Build history of the part. All positions in model axes, mm. A direction names the side the tool comes from. Give positions to 0.01 mm unless a question says otherwise; leave off trailing zeros. Order: outer loops, then holes, each group sorted by start corner. A loop starts at its lowest first (then second) coordinate and runs counter-clockwise, first axis right, second up. Notation, with made-up numbers: M 64.5,43.25 L 74.5,43.25 A5 cw 74.5,51.25 Z; hole C 44,80.5 d9. An arc over 180 degrees is marked long. Use CSV: the item, a comma, the result in double quotes. Start each with the question number.
Item 1: Band-saw the part on C-C on y = 3.5. Write the cut outline in (x, z), plus the area to 3 significant figures.
Item 2: Band-saw the part on D-D on x = -10. Write the cut outline in (y, z), plus the area to 3 significant figures.
Item 3: Band-saw the part on B-B on x = 5. Write the cut outline in (y, z), plus the area to 3 significant figures.
Item 4: Two-plate mould, pull along X, no slides. Class faces 1 (the flat face through (0, 11, 2)), 2 (the cylindrical face through (-10.55, -2.97, 7.44)), 3 (the flat face through (11.45, 0, 4)): pulls with the +X half, pulls with the -X half, needs draft (parallel to the pull), parting line crosses it, or undercut.
Item 5: Pin check, flat tips, straight feed: P1, Ø2.5, axis at x = 4.5, y = 10.5, coming from the +Z side; P2, Ø5.5, axis at x = 4.5, y = 11, coming from the -Z side; P3, Ø0.6, axis at x = 5, z = 7.5, coming from the +Y side. Stop position of each tip, or through.
Item 6: Wall check: line 1 along X through (y, z) = (2.25, 5); line 2 along X through (y, z) = (-2.5, 5.25); line 3 along X through (y, z) = (-4.5, 5.5). Give the ranges that are in metal, low to high.
Item 7: Which spindle directions (+Z, -Z, +X, -X, +Y, -Y) get a long thin tool onto all of the face, cutting with end or side? Do faces 4 (the flat face through (11.65, 0, 4)), 5 (the flat face through (0, -14.25, 4)), 6 (the flat face through (0, 11, 6.3)). Say none if no direction does.
Item 8: Band-saw the part on A-A on z = 4.25. Write the cut outline in (x, y), plus the area to 3 significant figures.
from build123d import *

# Parameters (mm, degrees)
EXTRUDE_1_DEPTH     = 14.25
CUT_EXTRUDE_START   = -12.229513
CUT_EXTRUDE_1_DEPTH = 24.459026


with BuildPart() as part:
    # Эскиз1 → Бобышка-Вытянуть1 (new, symmetric)
    with BuildSketch(Plane(origin=(0, 0, 0), x_dir=(1, 0, 0), z_dir=(0, 1, 0))):
        with BuildLine():
            Line((-9.25, 0), (9.25, 0))
            ThreePointArc((9.25, 0), (11.371320344, -0.878679656), (12.25, -3))
            Line((12.25, -3), (12.25, -5))
            ThreePointArc((12.25, -5), (11.95, -5.3), (11.65, -5))
            Line((11.65, -5), (11.65, -3.1))
            ThreePointArc((11.65, -3.1), (11.55, -3), (11.45, -3.1))
            Line((11.45, -3.1), (11.45, -5.3))
            ThreePointArc((11.45, -5.3), (10.571320344, -7.421320344), (8.45, -8.3))
            Line((8.45, -8.3), (-8.45, -8.3))
            ThreePointArc((-8.45, -8.3), (-10.571320344, -7.421320344), (-11.45, -5.3))
            Line((-11.45, -5.3), (-11.45, -3.1))
            ThreePointArc((-11.45, -3.1), (-11.55, -3), (-11.65, -3.1))
            Line((-11.65, -3.1), (-11.65, -5))
            ThreePointArc((-11.65, -5), (-11.95, -5.3), (-12.25, -5))
            Line((-12.25, -5), (-12.25, -3))
            ThreePointArc((-12.25, -3), (-11.371320344, -0.878679656), (-9.25, 0))
        make_face()
    extrude(amount=EXTRUDE_1_DEPTH, both=True)

    # Эскиз2 → Вырез-Вытянуть1 (cut)
    with BuildSketch(Plane(origin=(0, 0, 0), x_dir=(0, 0, -1), z_dir=(1, 0, 0)).offset(CUT_EXTRUDE_START)):
        with BuildLine():
            Line((-6.3, 13.6), (-6.3, 8.4))
            ThreePointArc((-6.3, 8.4), (-6.490380592, 7.940380592), (-6.95, 7.75))
            Line((-6.95, 7.75), (-7.65, 7.75))
            ThreePointArc((-7.65, 7.75), (-8.109619408, 7.559619408), (-8.3, 7.1))
            Line((-8.3, 7.1), (-8.3, 14.25))
            Line((-8.3, 14.25), (-8.3, 15.25))
            Line((-8.3, 15.25), (0, 15.25))
            Line((0, 15.25), (0, 7.1))
            ThreePointArc((0, 7.1), (-0.190380592, 7.559619408), (-0.65, 7.75))
            Line((-0.65, 7.75), (-1.35, 7.75))
            ThreePointArc((-1.35, 7.75), (-1.809619408, 7.940380592), (-2, 8.4))
            Line((-2, 8.4), (-2, 13.6))
            ThreePointArc((-2, 13.6), (-2.190380592, 14.059619408), (-2.65, 14.25))
            Line((-2.65, 14.25), (-5.65, 14.25))
            ThreePointArc((-5.65, 14.25), (-6.109619408, 14.059619408), (-6.3, 13.6))
        make_face()
    extrude(amount=CUT_EXTRUDE_1_DEPTH, mode=Mode.SUBTRACT)


solid = part.part
Model answer:
1,outline,"M -12.25,3 A3 ccw -9.25,0 L 9.25,0 A3 ccw 12.25,3 L 12.25,5 A0.3 ccw 11.65,5 L 11.65,3.1 A0.1 cw 11.45,3.1 L 11.45,5.3 A3 ccw 8.45,8.3 L -8.45,8.3 A3 ccw -11.45,5.3 L -11.45,3.1 A0.1 cw -11.65,3.1 L -11.65,5 A0.3 ccw -12.25,5 Z"
1,area,"190 mm^2"
2,outline,"M -14.25,0.1 L 7.44,0.1 A0.65 ccw 7.75,0.65 L 7.75,1.35 A0.65 cw 8.4,2 L 13.6,2 A0.65 ccw 14.25,2.65 L 14.25,5.65 A0.65 ccw 13.6,6.3 L 8.4,6.3 A0.65 cw 7.75,6.95 L 7.75,7.65 A0.65 ccw 7.71,7.87 L -14.25,7.87 Z"
2,area,"199 mm^2"
3,outline,"M -14.25,0 L 7.1,0 A0.65 ccw 7.75,0.65 L 7.75,1.35 A0.65 cw 8.4,2 L 13.6,2 A0.65 ccw 14.25,2.65 L 14.25,5.65 A0.65 ccw 13.6,6.3 L 8.4,6.3 A0.65 cw 7.75,6.95 L 7.75,7.65 A0.65 ccw 7.1,8.3 L -14.25,8.3 Z"
3,area,"210 mm^2"
4,face 1,"needs draft"
4,face 2,"pulls with the -X half"
4,face 3,"undercut"
5,P1,"stops at z = 6.3"
5,P2,"stops at z = 1.98"
5,P3,"stops at y = 7.75"
6,line 1,"x = -12.25 to -11.65, -11.45 to 11.45, 11.65 to 12.25"
6,line 2,"x = -12.12 to -11.78, -11.45 to 11.45, 11.78 to 12.12"
6,line 3,"x = -11.44 to 11.44"
7,face 4,"+Z, +Y, -Y"
7,face 5,"+Z, -Z, +X, -X, -Y"
7,face 6,"+Z, +X, -X, +Y"
8,outline,"M -12.25,-14.25 L -11.65,-14.25 L -11.65,14.25 L -12.25,14.25 Z; M -11.45,-14.25 L 11.45,-14.25 L 11.45,14.25 L -11.45,14.25 Z; M 11.65,-14.25 L 12.25,-14.25 L 12.25,14.25 L 11.65,14.25 Z"
8,area,"687 mm^2"
